For this review, take the finished solid that the model builds, in its own axes (mm). Face numbers are marked on the shaded views. Give positions to 0.01 mm unless a question says otherwise; leave off trailing zeros. Order: outer loops, then holes, each group sorted by start corner. A loop starts at its lowest first (then second) coordinate and runs counter-clockwise, first axis right, second up. Notation, with made-up numbers: (71, 50) - (119, 50) arc R23 cw to (119, 72) - close; hole circle Ø6 at (3, 77). An arc over 180 degrees is marked (long way). One line per item, written item: value.
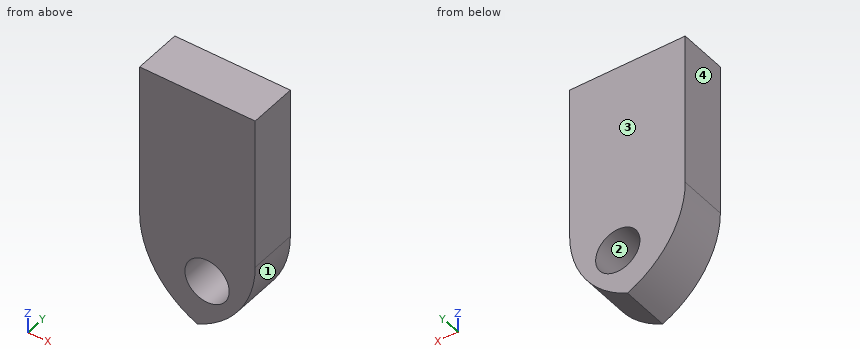
```python
from build123d import *

# Parameters (mm, degrees)
SKETCH1_W           = 7.62
SKETCH1_H           = 16.51
SKETCH1_R           = 1.4605
BOSS_EXTRUDE1_DEPTH = 3.175
FILLET3_R           = 6.35


with BuildPart() as part:
    # Sketch1 → Boss-Extrude1 (new body)
    with BuildSketch(Plane(origin=(0, 0, 0), x_dir=(1, 0, 0), z_dir=(0, 1, 0))):
        with Locations((3.81, 8.255)):
            Rectangle(SKETCH1_W, SKETCH1_H)
        with Locations(Location((4.445, 12.7, 0), (0, 0, 270))):
            Circle(SKETCH1_R, mode=Mode.SUBTRACT)
    extrude(amount=BOSS_EXTRUDE1_DEPTH)

    # Fillet3
    # the kernel refuses this fillet: 6.35 mm, written as the material it takes off along each edge
    with BuildSketch(Plane(origin=(0, -15.875, -16.51), x_dir=(1, 0, 0), z_dir=(0, 1, 0)), Plane(origin=(7.62, -15.875, -16.51), x_dir=(0, 0, 1), z_dir=(0, 1, 0))) as fillet3_piece_1:
        with BuildLine():
            CenterArc((FILLET3_R, -FILLET3_R), FILLET3_R, 90, 90)
            Line((0, -FILLET3_R), (0, 0))
            Line((0, 0), (FILLET3_R, 0))
        make_face()
    extrude(amount=34.925, mode=Mode.SUBTRACT)


solid = part.part
```
(1) Take a section at A-A (x = 5.25). Write out the cut boundary in (y, z) (3 decimals), then the cut area to 3 significant figures.
Answers below:
outline: (0, -15.108) - (3.175, -15.108) - (3.175, -13.919) - (0, -13.919) - close; (0, -11.481) - (3.175, -11.481) - (3.175, 0) - (0, 0) - close
area: 40.2 mm^2
(2) Take a section at B-B (z = -11.5). Write out the cut boundary in (x, y) (1 decimal).
Answers below:
outline: (0.1, 0) - (3.6, 0) - (3.6, 3.2) - (0.1, 3.2) - close; (5.3, 0) - (7.5, 0) - (7.5, 3.2) - (5.3, 3.2) - close
(3) Wall thickness on line 1 (Z direction, x = 3.25, y = 0.2); line 2 (Z direction, x = 5.25, y = 3); line 3 (X direction, y = 1.3, z = -12.7): over which ranges is each line inside the solid? List them lowest first. Write a range as from..to.
Answers below:
line 1: z = -15.7..-13.54, -11.86..0
line 2: z = -15.11..-13.92, -11.48..0
line 3: x = 0.53..2.98, 5.91..7.09
(4) Take a section at D-D (x = 2.75). Write out the cut boundary in (y, z) (3 decimals).
Answers below:
outline: (0, -15.391) - (3.175, -15.391) - (3.175, 0) - (0, 0) - close
(5) Draft analysis for pull direction X (two halves, no side actions). For the marked faces 1, 2, 3 and 4, state which applies: pulls with the +X half, pulls with the -X half, needs draft (parallel to the pull), parting line crosses it, or undercut.
Answers below:
face 1: pulls with the +X half
face 2: undercut
face 3: needs draft
face 4: pulls with the -X half
